from build123d import *

# Parameters (mm, degrees)
SHELL1_OUTLINE_R = 79.375
SHELL1_DEPTH     = 31.75


# Read off the part's stored shape, not the designer's step: Shell1
with BuildPart() as part:
    # Sketch1 → Revolve1 (revolve)
    with BuildSketch(Plane.XY, mode=Mode.PRIVATE) as revolve1_sk:
        Polygon((0, 0), (92.075, 0), (92.075, 19.05), (95.25, 19.05), (95.25, 44.45), (0, 44.45), align=None)
    revolve(revolve1_sk.sketch.rotate(Axis((0, 0, 0), (0, 1, 0)), 90), axis=Axis((0, 0, 0), (0, 1, 0)))

    # Shell1 outline → Shell1 (cut)
    with BuildSketch(Plane(origin=(0, 0, 0), x_dir=(1, 0, 0), z_dir=(0, 1, 0))):
        Circle(SHELL1_OUTLINE_R)
    extrude(amount=SHELL1_DEPTH, mode=Mode.SUBTRACT)


solid = part.part
Read the model definition and answer for the solid it produces. Units are mm, in the model's axes. A direction names the side the tool comes from. Round coordinates to 2 decimals unless told otherwise and drop trailing zeros. Order: outer loops, then holes, each group sorted by start corner. A loop starts at its lowest first (then second) coordinate and runs counter-clockwise, first axis right, second up.
1) Flat-ended cylindrical pins translate along their axes: pin 1 (1.5 mm diameter, centred on x = -19.5, z = 28.5, fed in from -Y); pin 2 (1.5 mm diameter, centred on x = 58, y = 17.5, fed in from -Z); pin 3 (6 mm diameter, centred on y = 20.5, z = 23, fed in from -X). Find the tip coordinate at first contact, or state that the pin passes through.
2) The part is cut by section A-A on z = 0. Write down the section's boundary in (x, y) (3 decimals).
3) The mould has two halves that part along X. Classify faces 1 (the face through (92.985, 31.928, 20.648)), 2 (the face through (-1, 31.75, -1)), 3 (the face through (75.71, 15.65, -23.84)), 4 (the face through (-78, 19.05, -50)): released by +X, released by -X, zero draft, split by the parting line, or undercut.
4) For faces 5 (the face through (-69, 0, 40)), 6 (the face through (89.885, 9.658, 19.96)), determine the directions among +Z, -Z, +X, -X, +Y, -Y from which every point of the face is accessible in a straight line to the end or side of a thin tool.
5) Straight lines are drawn through the part: L1, parallel to X at y = 14, z = 0 (3 decimals); L2, parallel to Y at x = -47, z = 55.5; L3, parallel to Z at x = -44.5, y = 29.5. For each, find the intervals that lie inside material, in ascending order.
6) The part is cut by section B-B on x = 14.5. Write down the section's boundary in (y, z), plus the area to 3 significant figures.
7) The part is cut by section C-C on y = 29. Write down the section's boundary in (x, z) (3 decimals), plus the area to 3 significant figures.
8) The part is cut by section D-D on y = 39. Write down the section's boundary in (x, z), plus the area to 3 significant figures.
Resolved:
1. pin 1: stops at y = 31.75
1. pin 2: stops at z = -72.11
1. pin 3: stops at x = -93.13
2. outline: (-95.25, 19.05) - (-92.075, 19.05) - (-92.075, 0) - (-79.375, 0) - (-79.375, 31.75) - (79.375, 31.75) - (79.375, 0) - (92.075, 0) - (92.075, 19.05) - (95.25, 19.05) - (95.25, 44.45) - (-95.25, 44.45) - close
3. face 1: split by the parting line
3. face 2: undercut
3. face 3: undercut
3. face 4: zero draft
4. face 5: +Z, -Z, +X, -X, -Y
4. face 6: -Y
5. L1: x = -92.075 to -79.375, 79.375 to 92.075
5. L2: y = 31.75 to 44.45
5. L3: z = -84.22 to -65.73, 65.73 to 84.22
6. outline: (0, -90.93) - (19.05, -90.93) - (19.05, -94.14) - (44.45, -94.14) - (44.45, 94.14) - (19.05, 94.14) - (19.05, 90.93) - (0, 90.93) - (0, 78.04) - (31.75, 78.04) - (31.75, -78.04) - (0, -78.04) - close
6. area: 3,290 mm2
7. outline: circle Ø190.5 at (0, 0); hole circle Ø158.75 at (0, 0)
7. area: 8,710 mm2
8. outline: circle Ø190.5 at (0, 0)
8. area: 28,500 mm2
